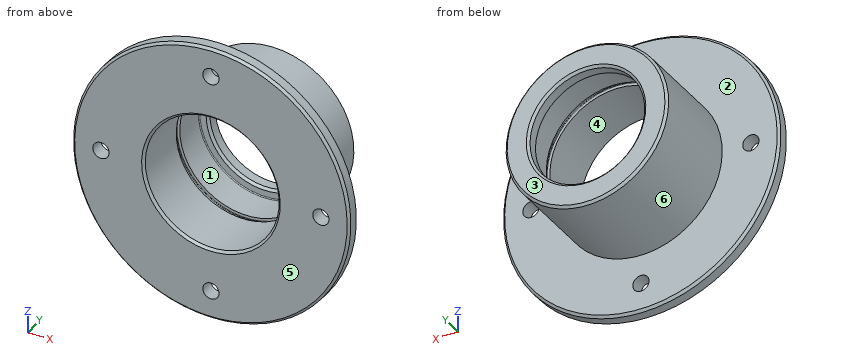
from build123d import *

# Parameters (mm, degrees)
M3_CLEARANCE_HOLE1_D = 3.4
FILLET1_R            = 0.2
CHAMFER1_SIZE        = 0.5


with BuildPart() as part:
    # Sketch1 → Revolve1 (revolve)
    with BuildSketch(Plane.XY, mode=Mode.PRIVATE) as revolve1_sk:
        Polygon((14, -3), (14, 17.15), (12, 17.15), (12, 20.15), (17, 20.15), (17, 0), (29, 0), (29, -3), align=None)
    revolve(revolve1_sk.sketch.rotate(Axis((0, 17.954019247, 0), (0, -1, 0)), 90), axis=Axis((0, 17.954019247, 0), (0, -1, 0)))

    # M3 Clearance Hole1 (through all)
    with Locations(Plane(origin=(0, 0, 0), x_dir=(1, 0, 0), z_dir=(0, 1, 0))):
        with Locations((0, 23), (23, 0), (0, -23), (-23, 0)):
            Hole(M3_CLEARANCE_HOLE1_D / 2)

    # Fillet1
    fillet1_edges = [part.edges().sort_by_distance(p)[0] for p in [
        (0, 17.15, -14),
    ]]
    fillet(fillet1_edges, radius=FILLET1_R)

    # Chamfer1
    chamfer1_edges = [part.edges().sort_by_distance(p)[0] for p in [
        (0, 17.15, -12),
        (0, 20.15, -12),
        (0, 20.15, -17),
        (0, 0, -29),
        (0, -3, -29),
        (0, -3, -14),
    ]]
    chamfer(chamfer1_edges, length=CHAMFER1_SIZE)

    # Sketch8 → Groove for BS 3673 P4 - B028M, Internal Circlip1 (revolve, cut)
    with BuildSketch(Plane(origin=(0, 17.954019247, 0), x_dir=(0, 0, 1), z_dir=(-1, 0, 0))):
        with BuildLine():
            Line((14.57, -9.104019247), (12.6, -9.104019247))
            Line((12.6, -9.104019247), (12.6, -7.804019247))
            Line((12.6, -7.804019247), (14.57, -7.804019247))
            ThreePointArc((14.57, -7.804019247), (14.661923882, -7.842095365), (14.7, -7.934019247))
            Line((14.7, -7.934019247), (14.7, -8.974019247))
            ThreePointArc((14.7, -8.974019247), (14.661923882, -9.065943128), (14.57, -9.104019247))
        make_face()
    revolve(axis=Axis((0, -32.045980753, 0), (0, 1, 0)), mode=Mode.SUBTRACT)


solid = part.part
Geometry check sheet. Reference: the model listing, model coordinates, mm. Face numbers are marked on the shaded views. A direction names the side the tool comes from. Coordinates: 2 decimals unless noted, no trailing zeros. Order: outer loops, then holes, each group sorted by start corner. A loop starts at its lowest first (then second) coordinate and runs counter-clockwise, first axis right, second up. Notation, with made-up numbers: (16, -8.5) -> (51, -8.5) arc R14 ccw to (51, -4.5) -> close; hole circle Ø6 at (20.25, 32). An arc over 180 degrees is marked (long way). Use a Markdown table: item, result. Add a question column.
1. Go/stop test with flat-tipped pins: pin 1 Ø3 at (y, z) = (8.5, 17) entering from -X; pin 2 Ø1 at (x, y) = (-1, 3.5) entering from -Z; pin 3 Ø8 at (x, z) = (-22, -10) entering from +Y. Record where each tip stops, or that it passes through.
2. Material ranges on L1, parallel to X at y = 9.45, z = 0; L2, parallel to X at y = 18.85, z = 0; L3, parallel to Y at x = 1, z = 19, recorded low to high.
3. Mould release check, pull along X, two halves, no side actions. Record for the marked faces 4, 5 and 6: pulls with the +X half, pulls with the -X half, needs draft (parallel to the pull), parting line crosses it, or undercut.
4. Set-up check for the marked faces 1, 2 and 3: record each of +Z, -Z, +X, -X, +Y, -Y from which the full face is reachable in a straight line by a thin tool's end or side.
5. Cross-section at A-A (x = 0). Give the number of separate pieces and of enclosed holes in the cut face, and give its area (3 significant figures).
6. Cross-section at C-C (y = 14.25). Enter the section's corners in (x, z), and give its area (3 significant figures).
Filled sheet:
| question | item | result |
|---|---|---|
| 1 | pin 1 | x = -6.98 |
| 1 | pin 2 | z = -16.99 |
| 1 | pin 3 | y = 0 |
| 2 | L1 | -17 to -14.7, 14.7 to 17 |
| 2 | L2 | -17 to -12, 12 to 17 |
| 2 | L3 | -3 to 0 |
| 3 | face 4 | undercut |
| 3 | face 5 | needs draft |
| 3 | face 6 | parting line crosses it |
| 4 | face 1 | -Y |
| 4 | face 2 | +Y |
| 4 | face 3 | +Z, -Z, +X, -X, +Y |
| 5 | separate pieces | 4 |
| 5 | enclosed holes | 0 |
| 5 | area | 199 mm2 |
| 6 | outline | circle Ø34 at (0, 0); hole circle Ø28 at (0, 0) |
| 6 | area | 292 mm2 |
